Build history of the part. All positions in model axes, mm. Face numbers are marked on the shaded views. Give positions to 0.01 mm unless a question says otherwise; leave off trailing zeros. Loops run counter-clockwise (first coordinate to the right, second up) from the corner with the lowest first, then second, coordinate; pieces in that order, holes last. Notation, with made-up numbers: (-24.75, -14) - (28.25, -14) arc R5 cw to (28.25, -5) - close; hole circle Ø7 at (59, 14). An arc over 180 degrees is marked (long way). Return JSON: item names as keys, results as strings. Group by question number.
1) Slice it at C-C (x = 38.1). List the corners of the cut face in (y, z), and give its area (3 significant figures).
2) Drill centre lines: probe 1 along Z at (x, y) = (38, -1); probe 2 along Z at (x, y) = (37.5, -5); probe 3 along X at (y, z) = (-6.75, 10). Where is each one in solid material? Low to high. Write a range as from..to.
3) Slice it at A-A (y = 0). List the corners of the cut face in (x, z).
4) Slice it at B-B (z = 9.75). List the corners of the cut face in (x, y), and give its area (3 significant figures).
5) Drop flat-ended pins along their axis: pin 1 (5 mm diameter, centred on x = 12.7, y = 0, fed in from -Z); pin 2 (3 mm diameter, centred on x = 26, z = 6.5, fed in from -Y). Give the stop position or say it passes through.
6) Mould opens along X. For the marked faces 1, 2, 3 and 4 say: released by +X, released by -X, zero draft, split by the parting line, or undercut.
7) Slice it at D-D (z = 6). List the corners of the cut face in (x, y).
```python
from build123d import *

# Parameters (mm, degrees)
SKETCH1_R           = 2.25
BOSS_EXTRUDE1_DEPTH = 22.2504
CUT_EXTRUDE1_REACH  = 57.683
SKETCH2_R           = 2.25
FILLET1_R           = 5
FILLET2_R           = 2


with BuildPart() as part:
    # Sketch1 → Boss-Extrude1 (new body)
    with BuildSketch(Plane.XY):
        Polygon((-6.35, -6.35), (31.75, -19.05), (44.45, -19.05), (44.45, 6.0452), (-6.35, 6.0452), align=None)
        with Locations(Location((0, 0, 0), (0, 0, 180))):
            Circle(SKETCH1_R, mode=Mode.SUBTRACT)
        with Locations(Location((12.7, 0, 0), (0, 0, 180))):
            Circle(SKETCH1_R, mode=Mode.SUBTRACT)
        with Locations(Location((25.4, 0, 0), (0, 0, 180))):
            Circle(SKETCH1_R, mode=Mode.SUBTRACT)
    extrude(amount=BOSS_EXTRUDE1_DEPTH)

    # Sketch2 → Cut-Extrude1 (cut, up to next)
    with BuildSketch(Plane(origin=(0, 6.0452, 0), x_dir=(1, 0, 0), z_dir=(0, 1, 0)), mode=Mode.PRIVATE) as cut_extrude1_sk1:
        with Locations(Location((38.1, -17.4752, 0), (0, 0, 270))):
            Circle(SKETCH2_R)
    cut_extrude1_tool1 = extrude(cut_extrude1_sk1.sketch, amount=-CUT_EXTRUDE1_REACH, mode=Mode.PRIVATE) & part.part
    # Sketch2 → Cut-Extrude1 (cut, up to next)
    with BuildSketch(Plane(origin=(0, 6.0452, 0), x_dir=(1, 0, 0), z_dir=(0, 1, 0)), mode=Mode.PRIVATE) as cut_extrude1_sk2:
        with Locations(Location((38.1, -4.7752, 0), (0, 0, 270))):
            Circle(SKETCH2_R)
    cut_extrude1_tool2 = extrude(cut_extrude1_sk2.sketch, amount=-CUT_EXTRUDE1_REACH, mode=Mode.PRIVATE) & part.part
    add(cut_extrude1_tool1.solids().sort_by_distance((38.1, 6.0452, 17.4752))[0], mode=Mode.SUBTRACT)
    add(cut_extrude1_tool2.solids().sort_by_distance((38.1, 6.0452, 4.7752))[0], mode=Mode.SUBTRACT)

    # Fillet1
    fillet1_edges = [part.edges().sort_by_distance(p)[0] for p in [
        (44.45, -6.5024, 0),
        (44.45, -6.5024, 22.2504),
        (31.75, -19.05, 11.1252),
        (-6.35, -6.35, 11.1252),
        (-6.35, 6.0452, 11.1252),
    ]]
    fillet(fillet1_edges, radius=FILLET1_R)

    # Fillet2
    fillet2_edges = [part.edges().sort_by_distance(p)[0] for p in [
        (36.00569415, -19.05, 0),
        (44.45, -19.05, 11.1252),
        (36.00569415, -19.05, 22.2504),
        (42.985533906, -19.05, 20.785933906),
        (42.985533906, -19.05, 1.464466094),
        (14.02455532, -13.14151844, 0),
        (-6.35, -0.85050195, 0),
        (19.05, 6.0452, 0),
        (-4.885533906, 4.580733906, 0),
        (-5.406210926, -5.669755323, 0),
        (31.760477086, -18.985437288, 0),
        (14.02455532, -13.14151844, 22.2504),
        (19.05, 6.0452, 22.2504),
        (-6.35, -0.85050195, 22.2504),
        (-4.885533906, 4.580733906, 22.2504),
        (-5.406210926, -5.669755323, 22.2504),
        (31.760477086, -18.985437288, 22.2504),
        (44.45, 6.0452, 11.1252),
        (42.985533906, 6.0452, 20.785933906),
        (42.985533906, 6.0452, 1.464466094),
    ]]
    fillet(fillet2_edges, radius=FILLET2_R)


solid = part.part
```
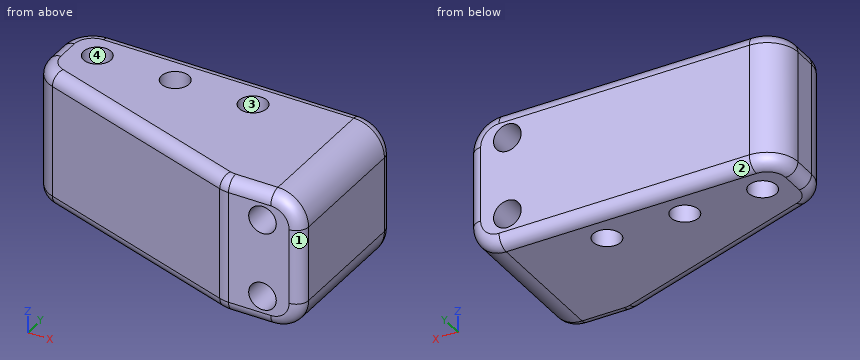
Results:
{
 "1": {"outline": "(-19.05, 2) arc R2 ccw to (-17.05, 0) - (4.05, 0) arc R2 ccw to (6.05, 2) - (6.05, 2.53) - (-19.05, 2.53) - close; (-19.05, 7.03) - (6.05, 7.03) - (6.05, 15.23) - (-19.05, 15.23) - close; (-19.05, 19.73) - (6.05, 19.73) - (6.05, 20.25) arc R2 ccw to (4.05, 22.25) - (-17.05, 22.25) arc R2 ccw to (-19.05, 20.25) - close", "area": "329 mm2"},
 "2": {"probe 1": "0..2.53, 7.02..15.23, 19.72..22.25", "probe 2": "0..2.61, 6.94..15.31, 19.64..22.25", "probe 3": "-4.34..44.45"},
 "3": {"outline": "(-6.35, 2) arc R2 ccw to (-4.35, 0) - (-2.25, 0) - (-2.25, 22.25) - (-4.35, 22.25) arc R2 ccw to (-6.35, 20.25) - close; (2.25, 0) - (10.45, 0) - (10.45, 22.25) - (2.25, 22.25) - close; (14.95, 0) - (23.15, 0) - (23.15, 22.25) - (14.95, 22.25) - close; (27.65, 0) - (39.45, 0) arc R5 ccw to (44.45, 5) - (44.45, 17.25) arc R5 ccw to (39.45, 22.25) - (27.65, 22.25) - close; hole circle Ø4.5 at (38.1, 4.78); hole circle Ø4.5 at (38.1, 17.48)"},
 "4": {"outline": "(-6.35, -2.75) arc R5 ccw to (-2.93, -7.49) - (30.98, -18.79) arc R5 ccw to (32.56, -19.05) - (42.45, -19.05) arc R2 ccw to (44.45, -17.05) - (44.45, 4.05) arc R2 ccw to (42.45, 6.05) - (-1.35, 6.05) arc R5 ccw to (-6.35, 1.05) - close; hole circle Ø4.5 at (0, 0); hole circle Ø4.5 at (12.7, 0); hole circle Ø4.5 at (25.4, 0)", "area": "976 mm2"},
 "5": {"pin 1": "z = 0", "pin 2": "y = -17.63"},
 "6": {"face 1": "released by +X", "face 2": "zero draft", "face 3": "undercut", "face 4": "undercut"},
 "7": {"outline": "(-6.35, -2.75) arc R5 ccw to (-2.93, -7.49) - (30.98, -18.79) arc R5 ccw to (32.56, -19.05) - (36.21, -19.05) - (36.21, 6.05) - (-1.35, 6.05) arc R5 ccw to (-6.35, 1.05) - close; (39.99, -19.05) - (42.45, -19.05) arc R2 ccw to (44.45, -17.05) - (44.45, 4.05) arc R2 ccw to (42.45, 6.05) - (39.99, 6.05) - close; hole circle Ø4.5 at (0, 0); hole circle Ø4.5 at (12.7, 0); hole circle Ø4.5 at (25.4, 0)"}
}
